The listing builds one solid part. Answer for the finished solid, in the listing's coordinates (mm). A direction names the side the tool comes from. Give positions to 0.01 mm unless a question says otherwise; leave off trailing zeros. Write each loop counter-clockwise with the first axis right and the second up, starting at its lowest first coordinate (ties: lowest second). Pieces come first, ordered by that corner, then holes. Notation, with made-up numbers: (-10, 48) - (48, 48) arc R27 ccw to (48, 65) - close; hole circle Ø9 at (32.5, -1.5). An arc over 180 degrees is marked (long way). Answer as CSV lines item,"result". Start each with the question number.
(1) For a pull along Y with two mould halves and no side action, classify faces 1 (the face through (0.3, 4.2, -0.1)), 2 (the face through (1.3, 0, 0)), 3 (the face through (9, 2, 0)) as pulls with the +Y half, pulls with the -Y half, needs draft (parallel to the pull), parting line crosses it, or undercut.
(2) Find section A-A (x = 1.75). Write down the section's boundary in (y, z), then the cut area to 3 significant figures.
(3) Straight lines are drawn through the part: probe 1 along Z at (x, y) = (6, 0.5); probe 2 along Z at (x, y) = (11.25, 1.5); probe 3 along X at (y, z) = (3.75, 1). For each, find the intervals that lie inside material, in ascending order.
(4) For faces 4 (the face through (1, -0.6, 0)), 5 (the face through (2.1, -0.78, 2.48)), determine the directions among +Z, -Z, +X, -X, +Y, -Y from which every point of the face is accessible in a straight line to the end or side of a thin tool.
(5) Each of these flat-tipped pins is pushed along its axis until it touches: pin 1 Ø1.5 at (x, y) = (11, 3) entering from +Z; pin 2 Ø1.5 at (x, y) = (10, 1.5) entering from +Z; pin 3 Ø1.4 at (x, z) = (0.5, 2) entering from -Y; pin 4 Ø3 at (x, y) = (12, -1) entering from -Z. Where does it stop, or does it pass through?
(6) Find section B-B (x = 7.25). Write down the section's boundary in (y, z).
from build123d import *

# Parameters (mm, degrees)
FILLET1_R  = 1
SKETCH2_W  = 8.4
SKETCH2_H  = 1.2
SLOT_DEPTH = 1.3


with BuildPart() as part:
    # BodySke → Base-Revolve (revolve)
    with BuildSketch(Plane.XY, mode=Mode.PRIVATE) as base_revolve_sk:
        Polygon((0, 0), (0, 4.2), (0.5, 4.2), (2.7, 2), (14, 2), (14, 0), align=None)
    revolve(base_revolve_sk.sketch.rotate(Axis((-6.35, 0, 0), (1, 0, 0)), 90), axis=Axis((-6.35, 0, 0), (1, 0, 0)))  # turned: the seam where the file's is

    # Fillet1
    fillet1_edges = [part.edges().sort_by_distance(p)[0] for p in [
        (2.7, 0, -2),
    ]]
    fillet(fillet1_edges, radius=FILLET1_R)

    # Sketch2 → Slot (cut)
    with BuildSketch(Plane.ZY):
        Rectangle(SKETCH2_W, SKETCH2_H)
    extrude(amount=-SLOT_DEPTH, mode=Mode.SUBTRACT)


solid = part.part
Result set:
1,face 1,"pulls with the +Y half"
1,face 2,"undercut"
1,face 3,"parting line crosses it"
2,outline,"circle Ø5.9 at (0, 0)"
2,area,"27.3 mm^2"
3,probe 1,"-1.94 to 1.94"
3,probe 2,"-1.32 to 1.32"
3,probe 3,"0 to 0.82"
4,face 4,"+Z, -Z, -X"
4,face 5,"+X"
5,pin 1,"through"
5,pin 2,"z = 1.85"
5,pin 3,"y = -3.99"
5,pin 4,"z = -2"
6,outline,"circle Ø4 at (0, 0)"
